```python
from build123d import *
from OCP.BRepFilletAPI import BRepFilletAPI_MakeChamfer

# Parameters (mm, degrees)
SKETCH_1_W               = 175
SKETCH_1_H               = 100
EXTRUDE_1_DEPTH          = 3
EXTRUDE_3_DEPTH          = 175
EXTRUDE_4_DEPTH          = 175
SKETCH_7_W               = 4.38851426
SKETCH_7_H               = 4.191593749
CUT_EXTRUDE_3_DEPTH      = 185.87600743
SKETCH_8_W               = 171
SKETCH_8_H               = 23.094010767
CUT_EXTRUDE_4_DEPTH      = 2
SKETCH_10_R              = 3.5
SKETCH_10_W              = 8
SKETCH_10_H              = 8
EXTRUDE_6_DEPTH          = 4
CUT_EXTRUDE_6_DEPTH      = 148.543018566
CUT_EXTRUDE_6_DEPTH_BACK = 148.543018566
SKETCH_2_R               = 1.4
SKETCH_11_W              = 145
SKETCH_11_H              = 12.237604307
CUT_EXTRUDE_7_DEPTH      = 23
SKETCH_13_W              = 4
SKETCH_13_H              = 4
CUT_EXTRUDE_8_DEPTH      = 148.283964791
CHAMFER_1_SIZE           = 1
CHAMFER_1_SIZE2          = 2.747477419
CUT_EXTRUDE_9_DEPTH      = 148.543018566
CUT_EXTRUDE_9_DEPTH_BACK = 148.543018566
SKETCH_15_W              = 48
SKETCH_15_H              = 40
SKETCH_15_W_2            = 9
SKETCH_15_H_2            = 15


with BuildPart() as part:
    # 草图1 → 凸台-拉伸1 (new body)
    with BuildSketch(Plane.XY):
        with Locations((-47.751936166, -7.814554894)):
            Rectangle(SKETCH_1_W, SKETCH_1_H)
    extrude(amount=EXTRUDE_1_DEPTH)

    # 草图3 → 凸台-拉伸3 (add, through all)
    with BuildSketch(Plane.ZY.offset(135.251936166)):
        Polygon((3, -57.814554894), (14.547005384, -57.814554894), (3, -37.814554894), align=None)
    extrude(amount=-EXTRUDE_3_DEPTH)

    # 草图5 → 凸台-拉伸4 (add, through all)
    with BuildSketch(Plane.ZY.offset(135.251936166)):
        Polygon((3, -37.814554894), (3, -34.814554894), (8.196152423, -34.814554894), align=None)
    extrude(amount=-EXTRUDE_4_DEPTH)

    # 草图7 → 切除-拉伸3 (cut, through all)
    with BuildSketch(Plane.ZY.offset(135.251936166)):
        with Locations((6.645542678, -35.647071791)):
            Rectangle(SKETCH_7_W, SKETCH_7_H)
    extrude(amount=-CUT_EXTRUDE_3_DEPTH, mode=Mode.SUBTRACT)

    # 草图8 → 切除-拉伸4 (cut)
    with BuildSketch(Plane(origin=(0, -8.154600618, -14.124182585), x_dir=(1, 0, 0), z_dir=(0, 0.49999999999999506, 0.8660254037844415))):
        with Locations((-47.751936166, -45.795370555)):
            Rectangle(SKETCH_8_W, SKETCH_8_H)
    extrude(amount=-CUT_EXTRUDE_4_DEPTH, mode=Mode.SUBTRACT)

    # 草图10 → 凸台-拉伸6 (add)
    with BuildSketch(Plane.XY.offset(3)):
        with Locations((-43.251936166, 32.185445106)):
            Circle(SKETCH_10_R)
        with Locations((14.748063834, 32.185445106)):
            Circle(SKETCH_10_R)
        with Locations((-43.251936166, -17.814554894)):
            Circle(SKETCH_10_R)
        with Locations((14.748063834, -17.814554894)):
            Circle(SKETCH_10_R)
        with Locations((-126.251936166, 34.685445106)):
            Rectangle(SKETCH_10_W, SKETCH_10_H)
        with Locations((30.748063834, 34.685445106)):
            Rectangle(SKETCH_10_W, SKETCH_10_H)
        with Locations((-126.251936166, 4.685445106)):
            Rectangle(SKETCH_10_W, SKETCH_10_H)
        with Locations((30.748063834, 4.685445106)):
            Rectangle(SKETCH_10_W, SKETCH_10_H)
    extrude(amount=EXTRUDE_6_DEPTH)

    # 草图2 → 切除-拉伸6 (cut, two sides: drawn at the far end of the back side and taken through both)
    with BuildSketch(Plane.XY.offset(3).offset(-CUT_EXTRUDE_6_DEPTH_BACK)):
        with Locations((-43.251936166, 32.185445106)):
            Circle(SKETCH_2_R)
        with Locations((14.748063834, 32.185445106)):
            Circle(SKETCH_2_R)
        with Locations((14.748063834, -17.814554894)):
            Circle(SKETCH_2_R)
        with Locations((-43.251936166, -17.814554894)):
            Circle(SKETCH_2_R)
    extrude(amount=CUT_EXTRUDE_6_DEPTH + CUT_EXTRUDE_6_DEPTH_BACK, mode=Mode.SUBTRACT)

    # 草图11 → 切除-拉伸7 (cut)
    with BuildSketch(Plane.XZ.offset(57.814554894)):
        with Locations((-47.751936166, 6.118802154)):
            Rectangle(SKETCH_11_W, SKETCH_11_H)
    extrude(amount=-CUT_EXTRUDE_7_DEPTH, mode=Mode.SUBTRACT)

    # 草图13 → 切除-拉伸8 (cut, through all)
    with BuildSketch(Plane.XY.offset(7)):
        with Locations((-126.251936166, 34.685445106)):
            Rectangle(SKETCH_13_W, SKETCH_13_H)
        with Locations((30.748063834, 34.685445106)):
            Rectangle(SKETCH_13_W, SKETCH_13_H)
        with Locations((-126.251936166, 4.685445106)):
            Rectangle(SKETCH_13_W, SKETCH_13_H)
        with Locations((30.748063834, 4.685445106)):
            Rectangle(SKETCH_13_W, SKETCH_13_H)
    extrude(amount=-CUT_EXTRUDE_8_DEPTH, mode=Mode.SUBTRACT)

    # 倒角1: one chamfer whose edges measure the first distance from different faces: ONE call of the kernel's chamfer builder (chamfer() names one face for all edges)
    chamfer_1_edges_1 = [part.edges().sort_by_distance(p)[0] for p in [
        (13.348063834, 32.185445106, 7),
    ]]
    chamfer_1_side_1 = [part.faces().sort_by_distance(p)[0] for p in [
        (11.347058783, 32.185445106, 7),
    ]]
    chamfer_1_edges_2 = [part.edges().sort_by_distance(p)[0] for p in [
        (-44.651936166, -17.814554894, 7),
    ]]
    chamfer_1_side_2 = [part.faces().sort_by_distance(p)[0] for p in [
        (-46.652941217, -17.814554894, 7),
    ]]
    chamfer_1_edges_3 = [part.edges().sort_by_distance(p)[0] for p in [
        (13.348063834, -17.814554894, 7),
    ]]
    chamfer_1_side_3 = [part.faces().sort_by_distance(p)[0] for p in [
        (11.347058783, -17.814554894, 7),
    ]]
    chamfer_1_edges_4 = [part.edges().sort_by_distance(p)[0] for p in [
        (-44.651936166, 32.185445106, 7),
    ]]
    chamfer_1_side_4 = [part.faces().sort_by_distance(p)[0] for p in [
        (-46.652941217, 32.185445106, 7),
    ]]
    chamfer_1_edges_5 = [part.edges().sort_by_distance(p)[0] for p in [
        (30.748063834, 36.685445106, 7),
        (28.748063834, 34.685445106, 7),
        (30.748063834, 32.685445106, 7),
        (32.748063834, 34.685445106, 7),
    ]]
    chamfer_1_side_5 = [part.faces().sort_by_distance(p)[0] for p in [
        (26.861200919, 34.685445106, 7),
    ]]
    chamfer_1_edges_6 = [part.edges().sort_by_distance(p)[0] for p in [
        (-126.251936166, 6.685445106, 7),
        (-128.251936166, 4.685445106, 7),
        (-126.251936166, 2.685445106, 7),
        (-124.251936166, 4.685445106, 7),
    ]]
    chamfer_1_side_6 = [part.faces().sort_by_distance(p)[0] for p in [
        (-130.138799081, 4.685445106, 7),
    ]]
    chamfer_1_edges_7 = [part.edges().sort_by_distance(p)[0] for p in [
        (30.748063834, 6.685445106, 7),
        (28.748063834, 4.685445106, 7),
        (30.748063834, 2.685445106, 7),
        (32.748063834, 4.685445106, 7),
    ]]
    chamfer_1_side_7 = [part.faces().sort_by_distance(p)[0] for p in [
        (26.861200919, 4.685445106, 7),
    ]]
    chamfer_1_edges_8 = [part.edges().sort_by_distance(p)[0] for p in [
        (-128.251936166, 34.685445106, 7),
        (-126.251936166, 32.685445106, 7),
        (-124.251936166, 34.685445106, 7),
        (-126.251936166, 36.685445106, 7),
    ]]
    chamfer_1_side_8 = [part.faces().sort_by_distance(p)[0] for p in [
        (-126.251936166, 38.572308021, 7),
    ]]
    chamfer_1 = BRepFilletAPI_MakeChamfer(part.part.solid().wrapped)
    for e in chamfer_1_edges_1:
        chamfer_1.Add(CHAMFER_1_SIZE, CHAMFER_1_SIZE2, e.wrapped, chamfer_1_side_1[0].wrapped)  # the first distance lies on this face
    for e in chamfer_1_edges_2:
        chamfer_1.Add(CHAMFER_1_SIZE, CHAMFER_1_SIZE2, e.wrapped, chamfer_1_side_2[0].wrapped)  # the first distance lies on this face
    for e in chamfer_1_edges_3:
        chamfer_1.Add(CHAMFER_1_SIZE, CHAMFER_1_SIZE2, e.wrapped, chamfer_1_side_3[0].wrapped)  # the first distance lies on this face
    for e in chamfer_1_edges_4:
        chamfer_1.Add(CHAMFER_1_SIZE, CHAMFER_1_SIZE2, e.wrapped, chamfer_1_side_4[0].wrapped)  # the first distance lies on this face
    for e in chamfer_1_edges_5:
        chamfer_1.Add(CHAMFER_1_SIZE, CHAMFER_1_SIZE2, e.wrapped, chamfer_1_side_5[0].wrapped)  # the first distance lies on this face
    for e in chamfer_1_edges_6:
        chamfer_1.Add(CHAMFER_1_SIZE, CHAMFER_1_SIZE2, e.wrapped, chamfer_1_side_6[0].wrapped)  # the first distance lies on this face
    for e in chamfer_1_edges_7:
        chamfer_1.Add(CHAMFER_1_SIZE, CHAMFER_1_SIZE2, e.wrapped, chamfer_1_side_7[0].wrapped)  # the first distance lies on this face
    for e in chamfer_1_edges_8:
        chamfer_1.Add(CHAMFER_1_SIZE, CHAMFER_1_SIZE2, e.wrapped, chamfer_1_side_8[0].wrapped)  # the first distance lies on this face
    add(Compound.cast(chamfer_1.Shape()), mode=Mode.REPLACE)

    # 草图15 → 切除-拉伸9 (cut, two sides: drawn at the far end of the back side and taken through both)
    with BuildSketch(Plane.XY.offset(3).offset(-CUT_EXTRUDE_9_DEPTH_BACK)):
        with Locations((-81.251936166, 7.185445106)):
            Rectangle(SKETCH_15_W, SKETCH_15_H)
        with Locations((-14.251936166, 7.185445106)):
            Rectangle(SKETCH_15_W, SKETCH_15_H)
        with Locations((-126.751936166, -48.314554894)):
            Rectangle(SKETCH_15_W_2, SKETCH_15_H_2)
        with Locations((31.248063834, -48.314554894)):
            Rectangle(SKETCH_15_W_2, SKETCH_15_H_2)
    extrude(amount=CUT_EXTRUDE_9_DEPTH + CUT_EXTRUDE_9_DEPTH_BACK, mode=Mode.SUBTRACT)


solid = part.part
```
CAD build for the part. Positions are in the model's coordinates, mm. A direction names the side the tool comes from. Coordinates: 2 decimals unless noted, no trailing zeros. Write each loop counter-clockwise with the first axis right and the second up, starting at its lowest first coordinate (ties: lowest second). Pieces come first, ordered by that corner, then holes. Notation, with made-up numbers: (21, 2) -> (75, 2) arc R14 cw to (75, 21) -> close; hole circle Ø5 at (60, -39.5). An arc over 180 degrees is marked (long way). Use CSV: the item, a comma, the result in double quotes. Start each with the question number.
Item 1: Band-saw the part on C-C, the plane y = -28. Write the cut outline in (x, z).
Item 2: Band-saw the part on B-B, the plane y = -4.5. Write the cut outline in (x, z), plus the area to 3 significant figures.
Item 3: Drop flat-ended pins along their axis: P1, Ø4.5, axis at x = -126.5, z = 6, coming from the +Y side; P2, Ø4.5, axis at x = 14.75, y = 32.19, coming from the -Z side; P3, Ø1.5, axis at y = -38.5, z = 5, coming from the -X side; P4, Ø4.5, axis at y = 6, z = 5.5, coming from the -X side. Give the stop position or say it passes through.
Item 4: Tool access for faces 1 (the flat face through (-126, 8.685, 5)), 2 (the flat face through (-122.252, 5, 5)), 3 (the flat face through (31, 38, 7)), 4 (the flat face through (37.748, -48, 8)), 5 (the flat face through (35.748, -50, 4)): list every direction of +Z, -Z, +X, -X, +Y, -Y with a clear straight run to the whole face (end or side of a thin tool).
Item 5: Wall check: probe 1 along X at (y, z) = (-43, 3); probe 2 along X at (y, z) = (1.5, 1); probe 3 along Z at (x, y) = (-92.5, -31.5). Give the ranges that are in metal, low to high.
Item 6: Band-saw the part on A-A, the plane x = -6.5. Write the cut outline in (y, z).
Item 7: Two-plate mould, pull along X, no slides. Class faces 6 (the conical face through (-44.921, 32.112, 4.996)), 7 (the flat face through (26.748, 35, 5)), 8 (the flat face through (-130.252, 35, 5)), 9 (the flat face through (-126, 38.685, 5)): +X half, -X half, draft (parallel to the pull), parting line (faces both ways), or undercut.
Response values:
1,outline,"(-135.25, 0) -> (39.75, 0) -> (39.75, 3) -> (-135.25, 3) -> close"
2,outline,"(-135.25, 0) -> (-105.25, 0) -> (-105.25, 3) -> (-135.25, 3) -> close; (-57.25, 0) -> (-38.25, 0) -> (-38.25, 3) -> (-57.25, 3) -> close; (9.75, 0) -> (39.75, 0) -> (39.75, 3) -> (9.75, 3) -> close"
2,area,"237 mm2"
3,P1,"stops at y = 38.69"
3,P2,"stops at z = 0"
3,P3,"passes through"
3,P4,"stops at x = -130.25"
4,face 1,"+Z, +X, -X"
4,face 2,"+Z, +Y"
4,face 3,"+Z, +X, -X, +Y"
4,face 4,"+Z"
4,face 5,"+Z, -Z"
5,probe 1,"x = -135.25 to -131.25, -122.25 to -120.25, 24.75 to 26.75, 35.75 to 39.75"
5,probe 2,"x = -135.25 to -105.25, -57.25 to -38.25, 9.75 to 39.75"
5,probe 3,"z = 0 to 3"
6,outline,"(-34.81, 0) -> (-12.81, 0) -> (-12.81, 3) -> (-34.81, 3) -> close; (27.19, 0) -> (42.19, 0) -> (42.19, 3) -> (27.19, 3) -> close"
7,face 6,"undercut"
7,face 7,"undercut"
7,face 8,"-X half"
7,face 9,"draft"
